Build history of the part. All positions in model axes, mm. Face numbers are marked on the shaded views. A direction names the side the tool comes from. Coordinates: 2 decimals unless noted, no trailing zeros. Order: outer loops, then holes, each group sorted by start corner. A loop starts at its lowest first (then second) coordinate and runs counter-clockwise, first axis right, second up. Notation, with made-up numbers: (-17, 55.5) - (19, 55.5) arc R19 cw to (19, 76.5) - close; hole circle Ø1 at (13, 57). An arc over 180 degrees is marked (long way). Answer as CSV lines item,"result". Start each with the question number.
from build123d import *

# Parameters (mm, degrees)
BOSS_EXTRUDE1_DEPTH = 2.5
FILLET1_R           = 5
SKETCH2_W           = 93
SKETCH2_H           = 50
BOSS_EXTRUDE2_DEPTH = 77
SKETCH8_R           = 2.660141884
SKETCH8_W           = 32
SKETCH8_H           = 35
SKETCH8_W_2         = 14.2
SKETCH8_H_2         = 7
SKETCH8_W_3         = 12.6
SKETCH8_H_3         = 19.5
CUT_EXTRUDE3_DEPTH  = 10
BOSS_EXTRUDE4_START = 5
SKETCH9_R           = 3.660141884
SKETCH9_R_2         = 2.660141884
SKETCH9_W           = 16.2
SKETCH9_H           = 9
SKETCH9_W_2         = 14.2
SKETCH9_H_2         = 7
BOSS_EXTRUDE4_DEPTH = 5
SKETCH10_W          = 5
SKETCH10_H          = 5
BOSS_EXTRUDE5_DEPTH = 10
SKETCH11_W          = 93
SKETCH11_H          = 50
BOSS_EXTRUDE6_DEPTH = 2.5
CUT_EXTRUDE4_REACH  = 101.36
SKETCH12_R          = 1.15


with BuildPart() as part:
    # Sketch1 → Boss-Extrude1 (new body)
    with BuildSketch(Plane(origin=(0, 0, 0), x_dir=(1, 0, 0), z_dir=(0, 1, 0))):
        with BuildLine():
            Line((-46.5, 30), (46.5, 30))
            ThreePointArc((46.5, 30), (50.035533906, 28.535533906), (51.5, 25))
            Line((51.5, 25), (51.5, -25))
            ThreePointArc((51.5, -25), (50.035533906, -28.535533906), (46.5, -30))
            Line((46.5, -30), (-46.5, -30))
            ThreePointArc((-46.5, -30), (-50.035533906, -28.535533906), (-51.5, -25))
            Line((-51.5, -25), (-51.5, 25))
            ThreePointArc((-51.5, 25), (-50.035533906, 28.535533906), (-46.5, 30))
        make_face()
    extrude(amount=BOSS_EXTRUDE1_DEPTH)

    # Fillet1
    # the kernel refuses this fillet: 5 mm, written as the material it takes off along each edge
    with BuildSketch(Plane(origin=(-46.5, 2.5, -25), x_dir=(-1, 0, 0), z_dir=(0, 0, 1))) as fillet1_piece_1:
        with BuildLine():
            CenterArc((0.669872981, 5), FILLET1_R, 270, 60)
            Line((0.669872981, 0), (0.669872981, -0.1))
            Line((0.669872981, -0.1), (5, -0.1))
            Line((5, -0.1), (5.1, 0))
            ThreePointArc((5.1, 0), (5.1, 1.25), (5.08660254, 2.45))
            Line((5.08660254, 2.45), (5, 2.5))
        make_face()
    revolve(axis=Axis((-46.5, 2.5, -25), (0, -1, 0)), revolution_arc=90, mode=Mode.SUBTRACT)
    with BuildSketch(Plane(origin=(-46.5, 2.5, -30), x_dir=(0, -1, 0), z_dir=(1, 0, 0)), Plane(origin=(46.5, 2.5, 30), x_dir=(0, -1, 0), z_dir=(-1, 0, 0))) as fillet1_piece_2:
        with BuildLine():
            CenterArc((5, -4.330127019), FILLET1_R, 120, 60)
            Line((0, -4.330127019), (-0.1, -4.330127019))
            Line((-0.1, -4.330127019), (-0.1, 0))
            Line((-0.1, 0), (0, 0.1))
            ThreePointArc((0, 0.1), (1.25, 0.1), (2.45, 0.08660254))
            Line((2.45, 0.08660254), (2.5, 0))
        make_face()
    extrude(amount=93, mode=Mode.SUBTRACT)
    with BuildSketch(Plane(origin=(46.5, 2.5, -25), x_dir=(0, 0, -1), z_dir=(-1, 0, 0))) as fillet1_piece_3:
        with BuildLine():
            CenterArc((0.669872981, 5), FILLET1_R, 270, 60)
            Line((0.669872981, 0), (0.669872981, -0.1))
            Line((0.669872981, -0.1), (5, -0.1))
            Line((5, -0.1), (5.1, 0))
            ThreePointArc((5.1, 0), (5.1, 1.25), (5.08660254, 2.45))
            Line((5.08660254, 2.45), (5, 2.5))
        make_face()
    revolve(axis=Axis((46.5, 2.5, -25), (0, -1, 0)), revolution_arc=90, mode=Mode.SUBTRACT)
    with BuildSketch(Plane(origin=(51.5, 2.5, -25), x_dir=(0, -1, 0), z_dir=(0, 0, 1)), Plane(origin=(-51.5, 2.5, 25), x_dir=(0, -1, 0), z_dir=(0, 0, -1))) as fillet1_piece_4:
        with BuildLine():
            CenterArc((5, -4.330127019), FILLET1_R, 120, 60)
            Line((0, -4.330127019), (-0.1, -4.330127019))
            Line((-0.1, -4.330127019), (-0.1, 0))
            Line((-0.1, 0), (0, 0.1))
            ThreePointArc((0, 0.1), (1.25, 0.1), (2.45, 0.08660254))
            Line((2.45, 0.08660254), (2.5, 0))
        make_face()
    extrude(amount=50, mode=Mode.SUBTRACT)
    with BuildSketch(Plane(origin=(46.5, 2.5, 25), x_dir=(1, 0, 0), z_dir=(0, 0, -1))) as fillet1_piece_5:
        with BuildLine():
            CenterArc((0.669872981, 5), FILLET1_R, 270, 60)
            Line((0.669872981, 0), (0.669872981, -0.1))
            Line((0.669872981, -0.1), (5, -0.1))
            Line((5, -0.1), (5.1, 0))
            ThreePointArc((5.1, 0), (5.1, 1.25), (5.08660254, 2.45))
            Line((5.08660254, 2.45), (5, 2.5))
        make_face()
    revolve(axis=Axis((46.5, 2.5, 25), (0, -1, 0)), revolution_arc=90, mode=Mode.SUBTRACT)
    with BuildSketch(Plane(origin=(-46.5, 2.5, 25), x_dir=(0, 0, 1), z_dir=(1, 0, 0))) as fillet1_piece_6:
        with BuildLine():
            CenterArc((0.669872981, 5), FILLET1_R, 270, 60)
            Line((0.669872981, 0), (0.669872981, -0.1))
            Line((0.669872981, -0.1), (5, -0.1))
            Line((5, -0.1), (5.1, 0))
            ThreePointArc((5.1, 0), (5.1, 1.25), (5.08660254, 2.45))
            Line((5.08660254, 2.45), (5, 2.5))
        make_face()
    revolve(axis=Axis((-46.5, 2.5, 25), (0, -1, 0)), revolution_arc=90, mode=Mode.SUBTRACT)

    # Sketch2 → Boss-Extrude2 (add)
    with BuildSketch(Plane.XZ):
        with BuildLine():
            Line((48.5, -25), (48.5, 25))
            ThreePointArc((48.5, 25), (47.914213562, 26.414213562), (46.5, 27))
            Line((46.5, 27), (-46.5, 27))
            ThreePointArc((-46.5, 27), (-47.914213562, 26.414213562), (-48.5, 25))
            Line((-48.5, 25), (-48.5, -25))
            ThreePointArc((-48.5, -25), (-47.914213562, -26.414213562), (-46.5, -27))
            Line((-46.5, -27), (46.5, -27))
            ThreePointArc((46.5, -27), (47.914213562, -26.414213562), (48.5, -25))
        make_face()
        Rectangle(SKETCH2_W, SKETCH2_H, mode=Mode.SUBTRACT)
    extrude(amount=BOSS_EXTRUDE2_DEPTH)

    # Sketch8 → Cut-Extrude3 (cut)
    with BuildSketch(Plane.XZ):
        with Locations(Location((42.218517518, 14.706886542, 0), (0, 0, 270))):
            Circle(SKETCH8_R)
        with Locations((-19.181482482, 0)):
            Rectangle(SKETCH8_W, SKETCH8_H)
        with Locations((8.918517518, 14)):
            Rectangle(SKETCH8_W_2, SKETCH8_H_2)
        with Locations((28.118517518, 14)):
            Rectangle(SKETCH8_W_2, SKETCH8_H_2)
        with Locations((8.118517518, -4.25)):
            Rectangle(SKETCH8_W_3, SKETCH8_H_3)
        with Locations((27.318517518, -4.25)):
            Rectangle(SKETCH8_W_3, SKETCH8_H_3)
    extrude(amount=-CUT_EXTRUDE3_DEPTH, mode=Mode.SUBTRACT)

    # Sketch9 → Boss-Extrude4 (add)
    # profile 1 of 3: a face of its own
    with BuildSketch(Plane.XZ.offset(BOSS_EXTRUDE4_START)):
        with Locations(Location((42.218517518, 14.706886542, 0), (0, 0, 90))):
            Circle(SKETCH9_R)
        with Locations(Location((42.218517518, 14.706886542, 0), (0, 0, 270))):
            Circle(SKETCH9_R_2, mode=Mode.SUBTRACT)
    # profile 2 of 3: a face of its own
    with BuildSketch(Plane.XZ.offset(BOSS_EXTRUDE4_START)):
        with Locations((8.918517518, 14)):
            Rectangle(SKETCH9_W, SKETCH9_H)
        with Locations((8.918517518, 14)):
            Rectangle(SKETCH9_W_2, SKETCH9_H_2, mode=Mode.SUBTRACT)
    # profile 3 of 3: a face of its own
    with BuildSketch(Plane.XZ.offset(BOSS_EXTRUDE4_START)):
        with Locations((28.118517518, 14)):
            Rectangle(SKETCH9_W, SKETCH9_H)
        with Locations((28.118517518, 14)):
            Rectangle(SKETCH9_W_2, SKETCH9_H_2, mode=Mode.SUBTRACT)
    extrude(amount=-BOSS_EXTRUDE4_DEPTH)

    # Sketch10 → Boss-Extrude5 (add)
    with BuildSketch(Plane.XZ.offset(77)):
        with Locations((44, 22.5)):
            Rectangle(SKETCH10_W, SKETCH10_H)
        with Locations((-44, 22.5)):
            Rectangle(SKETCH10_W, SKETCH10_H)
        with Locations((-44, -22.5)):
            Rectangle(SKETCH10_W, SKETCH10_H)
        with Locations((44, -22.5)):
            Rectangle(SKETCH10_W, SKETCH10_H)
    extrude(amount=-BOSS_EXTRUDE5_DEPTH)

    # Sketch11 → Boss-Extrude6 (add)
    with BuildSketch(Plane.XZ.offset(77)):
        with BuildLine():
            Line((46.5, 27), (-46.5, 27))
            ThreePointArc((-46.5, 27), (-47.914213562, 26.414213562), (-48.5, 25))
            Line((-48.5, 25), (-48.5, -25))
            ThreePointArc((-48.5, -25), (-47.914213562, -26.414213562), (-46.5, -27))
            Line((-46.5, -27), (46.5, -27))
            ThreePointArc((46.5, -27), (47.914213562, -26.414213562), (48.5, -25))
            Line((48.5, -25), (48.5, 25))
            ThreePointArc((48.5, 25), (47.914213562, 26.414213562), (46.5, 27))
        make_face()
        Rectangle(SKETCH11_W, SKETCH11_H, mode=Mode.SUBTRACT)
    extrude(amount=BOSS_EXTRUDE6_DEPTH)

    # Sketch12 → Cut-Extrude4 (cut, up to next)
    with BuildSketch(Plane.XZ.offset(77), mode=Mode.PRIVATE) as cut_extrude4_sk1:
        with Locations(Location((-44, 22.5, 0), (0, 0, 270))):
            Circle(SKETCH12_R)
    cut_extrude4_tool1 = extrude(cut_extrude4_sk1.sketch, amount=-CUT_EXTRUDE4_REACH, mode=Mode.PRIVATE) & part.part
    # Sketch12 → Cut-Extrude4 (cut, up to next)
    with BuildSketch(Plane.XZ.offset(77), mode=Mode.PRIVATE) as cut_extrude4_sk2:
        with Locations(Location((44, 22.5, 0), (0, 0, 270))):
            Circle(SKETCH12_R)
    cut_extrude4_tool2 = extrude(cut_extrude4_sk2.sketch, amount=-CUT_EXTRUDE4_REACH, mode=Mode.PRIVATE) & part.part
    # Sketch12 → Cut-Extrude4 (cut, up to next)
    with BuildSketch(Plane.XZ.offset(77), mode=Mode.PRIVATE) as cut_extrude4_sk3:
        with Locations(Location((44, -22.5, 0), (0, 0, 270))):
            Circle(SKETCH12_R)
    cut_extrude4_tool3 = extrude(cut_extrude4_sk3.sketch, amount=-CUT_EXTRUDE4_REACH, mode=Mode.PRIVATE) & part.part
    # Sketch12 → Cut-Extrude4 (cut, up to next)
    with BuildSketch(Plane.XZ.offset(77), mode=Mode.PRIVATE) as cut_extrude4_sk4:
        with Locations(Location((-44, -22.5, 0), (0, 0, 270))):
            Circle(SKETCH12_R)
    cut_extrude4_tool4 = extrude(cut_extrude4_sk4.sketch, amount=-CUT_EXTRUDE4_REACH, mode=Mode.PRIVATE) & part.part
    add(cut_extrude4_tool1.solids().sort_by_distance((-44, -77, 22.5))[0], mode=Mode.SUBTRACT)
    add(cut_extrude4_tool2.solids().sort_by_distance((44, -77, 22.5))[0], mode=Mode.SUBTRACT)
    add(cut_extrude4_tool3.solids().sort_by_distance((44, -77, -22.5))[0], mode=Mode.SUBTRACT)
    add(cut_extrude4_tool4.solids().sort_by_distance((-44, -77, -22.5))[0], mode=Mode.SUBTRACT)


solid = part.part
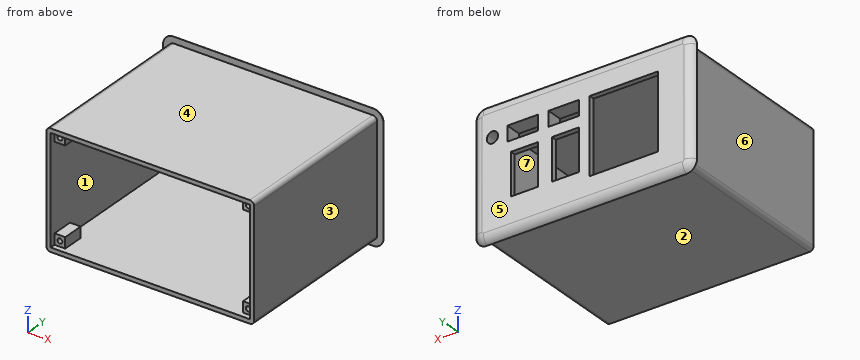
(1) Band-saw the part on C-C on x = 9. List the corners of the cut face in (y, z).
(2) Pull direction Z, two halves, no side cores. Call the marked faces 1, 2, 3 and 4: +Z half, -Z half, draft (parallel to the pull), parting line (faces both ways), or undercut.
(3) Which spindle directions (+Z, -Z, +X, -X, +Y, -Y) get a long thin tool onto all of the face, cutting with end or side? Do the marked faces 5, 6 and 7. Say none if no direction does.
(4) Band-saw the part on A-A on z = 0.5. List the corners of the cut face in (x, y), plus the area to 3 significant figures.
(5) Probe L1, parallel to X at y = -70.5, z = -22.5; L2, parallel to Z at x = -35.5, y = -35.5; L3, parallel to X at y = -18, z = 2. List the from-to ranges inside material, lowest first. Write a range as [from, to].
(6) Band-saw the part on B-B on y = -35.5. List the corners of the cut face in (x, z).
(7) Drop flat-ended pins along their axis: pin 1 Ø1.2 at (y, z) = (1, 0.5) entering from +X; pin 2 Ø2 at (y, z) = (-6.5, 6.5) entering from +X; pin 3 Ø1.5 at (y, z) = (-71, 22) entering from -X. Give the stop position or say it passes through.
(8) Band-saw the part on D-D on x = -38. List the corners of the cut face in (y, z), plus the area to 3 significant figures.
Filled in:
1,outline,"(-79.5, -27) - (0, -27) - (0, -30) arc R5 ccw to (2.5, -25.67) - (2.5, -14) - (0, -14) - (0, -25) - (-79.5, -25) - close; (-79.5, 25) - (0, 25) - (0, 18.5) - (-5, 18.5) - (-5, 17.5) - (2.5, 17.5) - (2.5, 25.67) arc R5 ccw to (0, 30) - (0, 27) - (-79.5, 27) - close; (-5, 9.5) - (0, 9.5) - (0, 5.5) - (2.5, 5.5) - (2.5, 10.5) - (-5, 10.5) - close"
2,face 1,"undercut"
2,face 2,"-Z half"
2,face 3,"draft"
2,face 4,"+Z half"
3,face 5,"+Z, -Z, +X, -X, +Y"
3,face 6,"+Z, -Z, -X, -Y"
3,face 7,"none"
4,outline,"(-51.5, 0) - (-48.5, 0) - (-48.5, -79.5) - (-46.5, -79.5) - (-46.5, 0) - (-35.18, 0) - (-35.18, 2.5) - (-47.17, 2.5) arc R5 ccw to start; (-3.18, 0) - (1.82, 0) - (1.82, 2.5) - (-3.18, 2.5) - close; (14.42, 0) - (21.02, 0) - (21.02, 2.5) - (14.42, 2.5) - close; (33.62, 0) - (46.5, 0) - (46.5, -79.5) - (48.5, -79.5) - (48.5, 0) - (51.5, 0) arc R5 ccw to (47.17, 2.5) - (33.62, 2.5) - close"
4,area,"426 mm^2"
5,L1,"x = [-48.5, -45.15], [-42.85, -41.5], [41.5, 42.85], [45.15, 48.5]"
5,L2,"z = [-27, -25], [25, 27]"
5,L3,"x = [-48.5, -46.5], [46.5, 48.5]"
6,outline,"(-48.5, -25) arc R2 ccw to (-46.5, -27) - (46.5, -27) arc R2 ccw to (48.5, -25) - (48.5, 25) arc R2 ccw to (46.5, 27) - (-46.5, 27) arc R2 ccw to (-48.5, 25) - close; hole (-46.5, -25) - (46.5, -25) - (46.5, 25) - (-46.5, 25) - close"
7,pin 1,"stops at x = 51.24"
7,pin 2,"stops at x = 48.5"
7,pin 3,"stops at x = -48.5"
8,outline,"(-79.5, -27) - (0, -27) - (0, -30) arc R5 ccw to (2.5, -25.67) - (2.5, 25.67) arc R5 ccw to (0, 30) - (0, 27) - (-79.5, 27) - (-79.5, 25) - (0, 25) - (0, -25) - (-79.5, -25) - close"
8,area,"462 mm^2"
